The listing builds one solid part. Answer for the finished solid, in the listing's coordinates (mm). Round coordinates to 2 decimals unless told otherwise and drop trailing zeros. Loops run counter-clockwise (first coordinate to the right, second up) from the corner with the lowest first, then second, coordinate; pieces in that order, holes last. Notation, with made-up numbers: (-2, 7) - (16, 7) arc R17 cw to (16, 21) - close; hole circle Ø1 at (-21, -28). An arc over 180 degrees is marked (long way). Write item = value, one per line. Start each with the question number.
1) For a pull along Y with two mould halves and no side action, classify faces 1 (the flat face through (-2.54, -1, 1)), 2 (the cylindrical face through (5.014, 5.586, 0.789)), 3 (the cylindrical face through (-0.01, 12.19, 0.79)) as released by +Y, released by -Y, zero draft, split by the parting line, or undercut.
2) Straight lines are drawn through the part: line 1 along X through (y, z) = (2.54, 1.2); line 2 along Y through (x, z) = (5.08, 0.3); line 3 along X through (y, z) = (8, 1.25). For each, find the intervals that lie inside material, in ascending order.
3) Section A-A, the plane y = 10.16 is taken. Determine the outline of the cut face in (x, z).
4) Section D-D, the plane x = -0.25 is taken. Determine the outline of the cut face in (y, z).
5) Section C-C, the plane z = 1.4 is taken. Give the number of separate pieces and of enclosed holes in the cut face, and give its area (3 significant figures).
6) Section B-B, the plane x = 5.08 is taken. Determine the outline of the cut face in (y, z).
from build123d import *

# Parameters (mm, degrees)
SKETCH_W             = 5.08
SKETCH_H             = 5.08
PAD_DEPTH            = 1.6
SKETCH001_R          = 0.51
POCKET_DEPTH         = 0.001
POCKET_DEPTH_BACK    = 1.601
POCKET001_DEPTH      = 1.601
POCKET001_DEPTH_BACK = 0.001
POCKET002_DEPTH      = 0.001
POCKET002_DEPTH_BACK = 1.601
ARRAY_X_COUNT        = 2
ARRAY_X_PITCH        = 5.08
ARRAY_Y_COUNT        = 3
ARRAY_Y_PITCH        = 5.08


with BuildPart() as part:
    # Sketch → Pad (new body)
    with BuildSketch(Plane.XY):
        Rectangle(SKETCH_W, SKETCH_H)
    extrude(amount=PAD_DEPTH)

    # Sketch001 → Pocket (cut, two sides)
    with BuildSketch(Plane.XY) as pocket_sk:
        Circle(SKETCH001_R)
    extrude(amount=-POCKET_DEPTH, mode=Mode.SUBTRACT)
    extrude(pocket_sk.sketch, amount=POCKET_DEPTH_BACK, mode=Mode.SUBTRACT)

    # Sketch002 → Pocket001 (cut, two sides)
    with BuildSketch(Plane.XY) as pocket001_sk:
        with BuildLine():
            ThreePointArc((-2.54, 2.03), (-2.179376, 2.179376), (-2.03, 2.54))
            Line((-2.54, 2.54), (-2.03, 2.54))
            Line((-2.54, 2.03), (-2.54, 2.54))
        make_face()
        with BuildLine():
            ThreePointArc((2.03, 2.54), (2.179376, 2.179376), (2.54, 2.03))
            Line((2.54, 2.54), (2.54, 2.03))
            Line((2.03, 2.54), (2.54, 2.54))
        make_face()
        with BuildLine():
            ThreePointArc((2.54, -2.03), (2.179376, -2.179376), (2.03, -2.54))
            Line((2.54, -2.54), (2.03, -2.54))
            Line((2.54, -2.03), (2.54, -2.54))
        make_face()
        with BuildLine():
            ThreePointArc((-2.03, -2.54), (-2.179376, -2.179376), (-2.54, -2.03))
            Line((-2.54, -2.54), (-2.54, -2.03))
            Line((-2.03, -2.54), (-2.54, -2.54))
        make_face()
    extrude(amount=POCKET001_DEPTH, mode=Mode.SUBTRACT)
    extrude(pocket001_sk.sketch, amount=-POCKET001_DEPTH_BACK, mode=Mode.SUBTRACT)

    # Sketch003 → Pocket002 (cut, two sides)
    with BuildSketch(Plane.XY) as pocket002_sk:
        with BuildLine():
            ThreePointArc((-0.51, 2.54), (0, 2.03), (0.51, 2.54))
            Line((0, 2.54), (0.51, 2.54))
            Line((-0.51, 2.54), (0, 2.54))
        make_face()
        with BuildLine():
            ThreePointArc((2.54, 0.51), (2.03, 0), (2.54, -0.51))
            Line((2.54, 0), (2.54, -0.51))
            Line((2.54, 0.51), (2.54, 0))
        make_face()
        with BuildLine():
            ThreePointArc((0.51, -2.54), (0, -2.03), (-0.51, -2.54))
            Line((0, -2.54), (-0.51, -2.54))
            Line((0.51, -2.54), (0, -2.54))
        make_face()
        with BuildLine():
            ThreePointArc((-2.54, -0.51), (-2.03, 0), (-2.54, 0.51))
            Line((-2.54, 0), (-2.54, 0.51))
            Line((-2.54, -0.51), (-2.54, 0))
        make_face()
    extrude(amount=-POCKET002_DEPTH, mode=Mode.SUBTRACT)
    extrude(pocket002_sk.sketch, amount=POCKET002_DEPTH_BACK, mode=Mode.SUBTRACT)

    # Array X: part ×2


with BuildPart() as part_1:
    add(part.part)
    with Locations(*[(i * ARRAY_X_PITCH, 0, 0) for i in range(1, ARRAY_X_COUNT)]):
        add(part.part)

    # Array Y: part ×3


with BuildPart() as part_2:
    add(part_1.part)
    with Locations(*[(0, i * ARRAY_Y_PITCH, 0) for i in range(1, ARRAY_Y_COUNT)]):
        add(part_1.part)


solid = part_2.part
Geometry check:
q1.face_1 = zero draft
q1.face_2 = undercut
q1.face_3 = released by +Y
q2.line_1 = -2.03 to -0.51, 0.51 to 2.03, 3.05 to 4.57, 5.59 to 7.11
q2.line_2 = -2.03 to -0.51, 0.51 to 2.03, 3.05 to 4.57, 5.59 to 7.11, 8.13 to 9.65, 10.67 to 12.19
q2.line_3 = -2.2 to -0.34, 0.34 to 2.2, 2.88 to 4.74, 5.42 to 7.28
q3.outline = (-2.03, 0) - (-0.51, 0) - (-0.51, 1.6) - (-2.03, 1.6) - close; (0.51, 0) - (2.03, 0) - (2.03, 1.6) - (0.51, 1.6) - close; (3.05, 0) - (4.57, 0) - (4.57, 1.6) - (3.05, 1.6) - close; (5.59, 0) - (7.11, 0) - (7.11, 1.6) - (5.59, 1.6) - close
q4.outline = (-2.1, 0) - (-0.44, 0) - (-0.44, 1.6) - (-2.1, 1.6) - close; (0.44, 0) - (2.1, 0) - (2.1, 1.6) - (0.44, 1.6) - close; (2.98, 0) - (4.64, 0) - (4.64, 1.6) - (2.98, 1.6) - close; (5.52, 0) - (7.18, 0) - (7.18, 1.6) - (5.52, 1.6) - close; (8.06, 0) - (9.72, 0) - (9.72, 1.6) - (8.06, 1.6) - close; (10.6, 0) - (12.26, 0) - (12.26, 1.6) - (10.6, 1.6) - close
q5.separate_pieces = 1
q5.enclosed_holes = 15
q5.area = 135 mm2
q6.outline = (-2.03, 0) - (-0.51, 0) - (-0.51, 1.6) - (-2.03, 1.6) - close; (0.51, 0) - (2.03, 0) - (2.03, 1.6) - (0.51, 1.6) - close; (3.05, 0) - (4.57, 0) - (4.57, 1.6) - (3.05, 1.6) - close; (5.59, 0) - (7.11, 0) - (7.11, 1.6) - (5.59, 1.6) - close; (8.13, 0) - (9.65, 0) - (9.65, 1.6) - (8.13, 1.6) - close; (10.67, 0) - (12.19, 0) - (12.19, 1.6) - (10.67, 1.6) - close
